The model under review builds one solid part; all positions refer to its coordinate system, in mm. Give positions to 0.01 mm unless a question says otherwise; leave off trailing zeros. Loops run counter-clockwise (first coordinate to the right, second up) from the corner with the lowest first, then second, coordinate; pieces in that order, holes last. Notation, with made-up numbers: M 47.25,69 L 97.25,69 A28 ccw 97.25,94 Z; hole C -10,-31 d10. An arc over 180 degrees is marked long. Put each result on its own line as item: value. Start each with the question number.
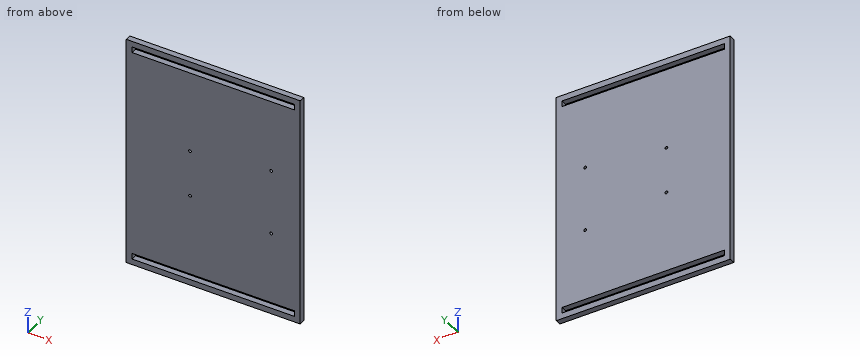
```python
from build123d import *

# Parameters (mm, degrees)
SKETCH1_W           = 150
SKETCH1_H           = 200
BOSS_EXTRUDE1_DEPTH = 100
SHELL2_T            = -5
SKETCH5_R           = 1.9
CUT_EXTRUDE2_DEPTH  = 10
BOSS_EXTRUDE4_DEPTH = 200
SKETCH9_W           = 101.133931545
SKETCH9_H           = 31.996148617
CUT_EXTRUDE4_DEPTH  = 236.849528301
SKETCH10_R          = 4
CUT_EXTRUDE5_DEPTH  = 10
CUT_EXTRUDE7_REACH  = 162.078
SKETCH11_W          = 140
SKETCH11_H          = 5
SKETCH15_R          = 1.2
CUT_EXTRUDE11_DEPTH = 10
SKETCH36_W          = 60
SKETCH36_H          = 5
BOSS_EXTRUDE7_DEPTH = 10
SKETCH37_R          = 3.5
CUT_EXTRUDE15_DEPTH = 60
SKETCH38_R          = 5
CUT_EXTRUDE16_DEPTH = 70
SKETCH39_W          = 156.49295795
SKETCH39_H          = 102.702702005
CUT_EXTRUDE17_DEPTH = 236.849528301


with BuildPart() as part:
    # Sketch1 → Boss-Extrude1 (new body)
    with BuildSketch(Plane(origin=(0, 0, 0), x_dir=(1, 0, 0), z_dir=(0, 1, 0))):
        Rectangle(SKETCH1_W, SKETCH1_H)
    extrude(amount=BOSS_EXTRUDE1_DEPTH)

    # Shell2
    shell2_openings = [part.faces().sort_by_distance(p)[0] for p in [
        (0, 50, -100),
        (0, 50, 100),
    ]]
    offset(amount=SHELL2_T, openings=shell2_openings, kind=Kind.INTERSECTION)

    # Sketch5 → Cut-Extrude2 (cut)
    with BuildSketch(Plane.XZ):
        with Locations(Location((-65, 91, 0), (0, 0, 270))):
            Circle(SKETCH5_R)
        with Locations(Location((-35, 91, 0), (0, 0, 270))):
            Circle(SKETCH5_R)
        with Locations(Location((-65, 67, 0), (0, 0, 270))):
            Circle(SKETCH5_R)
        with Locations(Location((-35, 67, 0), (0, 0, 270))):
            Circle(SKETCH5_R)
    cut_extrude2 = extrude(amount=-CUT_EXTRUDE2_DEPTH, mode=Mode.SUBTRACT)

    # Mirror2: Cut-Extrude2 across plane
    add(cut_extrude2.mirror(Plane.XY), mode=Mode.SUBTRACT)

    # Sketch8 → Boss-Extrude4 (add, through all)
    with BuildSketch(Plane.XY.offset(100)):
        Polygon((-15, 17), (75, 17), (75, 22), (-20, 22), (-20, 0), (-15, 0), align=None)
    extrude(amount=-BOSS_EXTRUDE4_DEPTH)

    # Sketch9 → Cut-Extrude4 (cut, through all)
    with BuildSketch(Plane.XY.offset(100)):
        with Locations((35.566965773, 1.001925691)):
            Rectangle(SKETCH9_W, SKETCH9_H)
    extrude(amount=-CUT_EXTRUDE4_DEPTH, mode=Mode.SUBTRACT)

    # Sketch10 → Cut-Extrude5 (cut)
    with BuildSketch(Plane.XZ.offset(-17)):
        with Locations((60, 0)):
            Circle(SKETCH10_R)
    extrude(amount=-CUT_EXTRUDE5_DEPTH, mode=Mode.SUBTRACT)

    # Cut-Extrude7: up to this face of the body (flat: up to its plane)
    cut_extrude7_end = Plane(part.part.faces().sort_by_distance((-44.954220044, 5, 0))[0])
    # Sketch11 → Cut-Extrude7 (cut, up to the picked face)
    with BuildSketch(Plane(origin=(0, 100, 0), x_dir=(1, 0, 0), z_dir=(0, 1, 0)), mode=Mode.PRIVATE) as cut_extrude7_sk1:
        with Locations((0, -92.5)):
            Rectangle(SKETCH11_W, SKETCH11_H)
    cut_extrude7_tool1 = split(extrude(cut_extrude7_sk1.sketch, amount=-CUT_EXTRUDE7_REACH, mode=Mode.PRIVATE), bisect_by=cut_extrude7_end, keep=Keep.BOTH, mode=Mode.PRIVATE)
    cut_extrude7 = cut_extrude7_tool1.solids().sort_by(Axis((0, 100, 92.5), (0, -1, 0)))[0]
    add(cut_extrude7, mode=Mode.SUBTRACT)

    # Mirror3: Cut-Extrude7 across plane
    add(cut_extrude7.mirror(Plane.XY), mode=Mode.SUBTRACT)

    # Sketch15 → Cut-Extrude11 (cut)
    with BuildSketch(Plane(origin=(0, 100, 0), x_dir=(1, 0, 0), z_dir=(0, 1, 0))):
        with Locations(Location((50, 28, 0), (0, 0, 270))):
            Circle(SKETCH15_R)
        with Locations(Location((50, -28, 0), (0, 0, 270))):
            Circle(SKETCH15_R)
        with Locations(Location((-20, 20, 0), (0, 0, 270))):
            Circle(SKETCH15_R)
        with Locations(Location((-20, -20, 0), (0, 0, 270))):
            Circle(SKETCH15_R)
    extrude(amount=-CUT_EXTRUDE11_DEPTH, mode=Mode.SUBTRACT)

    # Sketch36 → Boss-Extrude7 (add)
    with BuildSketch(Plane.ZY.offset(-70)):
        with Locations((-13.202053215, 62.5)):
            Rectangle(SKETCH36_W, SKETCH36_H)
    boss_extrude7 = extrude(amount=BOSS_EXTRUDE7_DEPTH)

    # Mirror5: Boss-Extrude7 across plane
    add(boss_extrude7.mirror(Plane(origin=(0, 0, 0), x_dir=(0, 0, 1), z_dir=(1, 0, 0))))

    # Sketch37 → Cut-Extrude15 (cut)
    with BuildSketch(Plane(origin=(75, 0, 0), x_dir=(0, 0, -1), z_dir=(1, 0, 0))):
        with Locations((0, 75)):
            Circle(SKETCH37_R)
    extrude(amount=-CUT_EXTRUDE15_DEPTH, mode=Mode.SUBTRACT)

    # Sketch38 → Cut-Extrude16 (cut)
    with BuildSketch(Plane.ZY.offset(75)):
        with Locations((0, 80)):
            Circle(SKETCH38_R)
    extrude(amount=-CUT_EXTRUDE16_DEPTH, mode=Mode.SUBTRACT)

    # Sketch39 → Cut-Extrude17 (cut, through all)
    with BuildSketch(Plane.XY.offset(100)):
        with Locations((3.246478975, 43.648648997)):
            Rectangle(SKETCH39_W, SKETCH39_H)
    extrude(amount=-CUT_EXTRUDE17_DEPTH, mode=Mode.SUBTRACT)


solid = part.part
```
Item 1: Consider section B-B, the plane x = 29.5. Write out the cut boundary in (y, z), plus the area to 3 significant figures.
Item 2: To check wall thickness, follow L1, parallel to Z at x = 8.5, y = 98.4; L2, parallel to X at y = 98.2, z = 28; L3, parallel to X at y = 98.55, z = -20. State the ranges of each line that lie inside material, in increasing order. Write a range as [from, to].
Item 3: Consider section A-A, the plane y = 98.1. Write out the cut boundary in (x, z), plus the area to 3 significant figures.
Report:
1. outline: M 95,-100 L 100,-100 L 100,-95 L 95,-95 Z; M 95,-90 L 100,-90 L 100,90 L 95,90 Z; M 95,95 L 100,95 L 100,100 L 95,100 Z
1. area: 950 mm²
2. L1: [-100, -95], [-90, 90], [95, 100]
2. L2: [-75, 48.8], [51.2, 75]
2. L3: [-75, -21.2], [-18.8, 75]
3. outline: M -75,-100 L 75,-100 L 75,100 L -75,100 Z; hole M -70,-95 L 70,-95 L 70,-90 L -70,-90 Z; hole M -70,90 L 70,90 L 70,95 L -70,95 Z; hole C -20,-20 d2.4; hole C -20,20 d2.4; hole C 50,-28 d2.4; hole C 50,28 d2.4
3. area: 28,600 mm²
